from build123d import *

# Parameters (mm, degrees)
CUT_EXTRUDE_1_REACH = 93.462
SKETCH_2_W          = 5
SKETCH_2_H          = 4.6
CUT_EXTRUDE_2_REACH = 93.462


with BuildPart() as part:
    # 草图1 → 旋转1 (revolve)
    with BuildSketch(Plane(origin=(0, 0, 0), x_dir=(1, 0, 0), z_dir=(0, 1, 0)), mode=Mode.PRIVATE) as revolve_1_sk:
        with BuildLine():
            Line((0, 10), (0, 14))
            Line((0, 14), (1.5, 14))
            Line((1.5, 14), (1.5, 24.75))
            Line((1.5, 24.75), (46.5, 24.75))
            Line((46.5, 24.75), (46.5, 22.5))
            Line((46.5, 22.5), (62.5, 22.5))
            Line((62.5, 22.5), (62.5, 21.25))
            Line((62.5, 21.25), (64.2, 21.25))
            Line((64.2, 21.25), (64.2, 22.5))
            Line((64.2, 22.5), (82.5, 22.5))
            ThreePointArc((82.5, 22.5), (83.914213562, 21.914213562), (84.5, 20.5))
            Line((84.5, 20.5), (84.5, 16))
            ThreePointArc((84.5, 16), (83.914213562, 14.585786438), (82.5, 14))
            Line((82.5, 14), (56.5, 14))
            Line((56.5, 14), (56.5, 14.25))
            Line((56.5, 14.25), (34.5, 14.25))
            Line((34.5, 14.25), (34.5, 18))
            Line((34.5, 18), (22.5, 18))
            Line((22.5, 18), (22.5, 10))
            Line((22.5, 10), (0, 10))
        make_face()
    revolve(revolve_1_sk.sketch.rotate(Axis((-32.624113475, 0, 0), (1, 0, 0)), 180), axis=Axis((-32.624113475, 0, 0), (1, 0, 0)))

    # 草图2 → 切除-拉伸1 (cut, up to next)
    with BuildSketch(Plane.ZY, mode=Mode.PRIVATE) as cut_extrude_1_sk1:
        with Locations((0, 10)):
            Rectangle(SKETCH_2_W, SKETCH_2_H)
    cut_extrude_1_tool1 = extrude(cut_extrude_1_sk1.sketch, amount=-CUT_EXTRUDE_1_REACH, mode=Mode.PRIVATE) & part.part
    add(cut_extrude_1_tool1.solids().sort_by_distance((0, 10, 0))[0], mode=Mode.SUBTRACT)

    # 草图3 → 切除-拉伸2 (cut, up to next)
    with BuildSketch(Plane(origin=(84.5, 0, 0), x_dir=(0, 0, -1), z_dir=(1, 0, 0)), mode=Mode.PRIVATE) as cut_extrude_2_sk1:
        Polygon((4, 14.7), (4, 10.868150386), (-4, 10.868150386), (-4, 14.7), (-4, 17.3), (4, 17.3), align=None)
    cut_extrude_2_tool1 = extrude(cut_extrude_2_sk1.sketch, amount=-CUT_EXTRUDE_2_REACH, mode=Mode.PRIVATE) & part.part
    add(cut_extrude_2_tool1.solids().sort_by_distance((84.5, 14.084075, 0))[0], mode=Mode.SUBTRACT)


solid = part.part
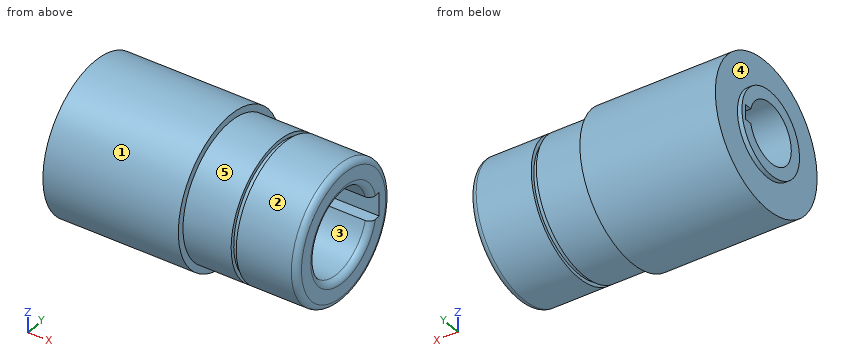
Model file for the job. Use its own axes, mm. Face numbers are marked on the shaded views. A direction names the side the tool comes from. Round coordinates to 2 decimals unless told otherwise and drop trailing zeros. Order: outer loops, then holes, each group sorted by start corner. A loop starts at its lowest first (then second) coordinate and runs counter-clockwise, first axis right, second up. Notation, with made-up numbers: M -33.75,17.5 L -15.75,17.5 A26 ccw -15.75,39.5 Z; hole C 57,40 d5. An arc over 180 degrees is marked long. Write each question's results on one line, items separated by ' | '. Start each with the question number.
(1) Saw through at A-A, the plane x = 38. Give the cut face in (y, z).
(2) Saw through at C-C, the plane x = 26.5. Give the cut face in (y, z).
(3) Probe probe 1 along Y at (x, z) = (52, 0); probe 2 along X at (y, z) = (9, -21.5); probe 3 along X at (y, z) = (-12, 12). List the from-to ranges inside material, lowest first. Write a range as from..to.
(4) Saw through at B-B, the plane x = 59.5. Give the cut face in (y, z), then the cut area to 3 significant figures.
(5) Drop flat-ended pins along their axis: pin 1 (1.5 mm diameter, centred on x = 69.5, y = 13.5, fed in from +Z); pin 2 (1.3 mm diameter, centred on x = 7.5, y = 11.5, fed in from +Z) (3 decimals); pin 3 (18 mm diameter, centred on y = -1, z = -7, fed in from +X); pin 4 (12 mm diameter, centred on x = 74.5, y = -17, fed in from -Z). Give the stop position or say it passes through.
(6) Which spindle directions (+Z, -Z, +X, -X, +Y, -Y) get a long thin tool onto all of the face, cutting with end or side? Do the marked faces 1 and 2. Say none if no direction does.
(7) Two-plate mould, pull along Z, no slides. Class the marked faces 3, 4 and 5: pulls with the +Z half, pulls with the -Z half, needs draft (parallel to the pull), parting line crosses it, or undercut.
Established:
1) outline: C 0,0 d49.5; hole M 13.68,-4 L 17.3,-4 L 17.3,4 L 13.68,4 A14.25 ccw long Z
2) outline: C 0,0 d49.5; hole C 0,0 d36
3) probe 1: y = -22.5..-14.25, 17.3..22.5 | probe 2: x = 1.5..46.5 | probe 3: x = 1.5..22.5, 34.5..84.5
4) outline: C 0,0 d45; hole M 13.42,-4 L 17.3,-4 L 17.3,4 L 13.42,4 A14 ccw long Z | area: 947 mm^2
5) pin 1: stops at z = 18.54 | pin 2: stops at z = 22.245 | pin 3: stops at x = 84.5 | pin 4: stops at z = -19.63
6) face 1: +X, -X | face 2: +X
7) face 3: undercut | face 4: needs draft | face 5: parting line crosses it
